```python
from build123d import *

# Parameters (mm, degrees)
F0_R     = 125
F2_DEPTH = 10
F1_R     = 15
F3_DEPTH = 10
F4_R     = 5
F5_R     = 9.544074
F6_DEPTH = 196


with BuildPart() as f2:
    # F0 (on Top) → F2 (new body)
    with BuildSketch(Plane.XY):
        Circle(F0_R)
    extrude(amount=-F2_DEPTH)

    # F1 (on face) → F3 (cut)
    with BuildSketch(Plane.XY):
        with Locations((-42.426407, 42.426407)):
            Circle(F1_R)
        with Locations((0, 60)):
            Circle(F1_R)
        with Locations((42.426407, 42.426407)):
            Circle(F1_R)
        with Locations((60, 0)):
            Circle(F1_R)
        with Locations((42.426407, -42.426407)):
            Circle(F1_R)
        with Locations((0, -60)):
            Circle(F1_R)
        with Locations((-42.426407, -42.426407)):
            Circle(F1_R)
        with Locations((-60, 0)):
            Circle(F1_R)
    extrude(amount=-F3_DEPTH, mode=Mode.SUBTRACT)

    # F4
    f4_edges = [f2.edges().sort_by_distance(p)[0] for p in [
        (-125, 0, 0),
    ]]
    fillet(f4_edges, radius=F4_R)

    # F5 (on face) → F6 (join)
    with BuildSketch(Plane(origin=(0, 0, -10), x_dir=(1, 0, 0), z_dir=(0, 0, -1))):
        with Locations((0, 105.908468)):
            Circle(F5_R)
        with Locations((104.299481, 18.390813)):
            Circle(F5_R)
        with Locations((36.22283, -99.521406)):
            Circle(F5_R)
        with Locations((-91.719424, -52.954234)):
            Circle(F5_R)
    extrude(amount=F6_DEPTH)


solid = f2.part
```
Part model, mm, in its own coordinate system. A direction names the side the tool comes from. Coordinates: 2 decimals unless noted, no trailing zeros. Order: outer loops, then holes, each group sorted by start corner. A loop starts at its lowest first (then second) coordinate and runs counter-clockwise, first axis right, second up. Notation, with made-up numbers: (84.5, 58) - (108.5, 58) arc R19 ccw to (108.5, 90) - close; hole circle Ø10 at (-37, -28.5). An arc over 180 degrees is marked (long way). Return JSON: item names as keys, results as strings. Group by question number.
Item 1: Which spindle directions (+Z, -Z, +X, -X, +Y, -Y) get a long thin tool onto all of the face, cutting with end or side? Do faces 1 (the face through (-2.1, -96.6, -106.6)), 2 (the face through (0, -106, -206)). Say none if no direction does.
Item 2: Cut at C-C (z = -149.5). List the corners of the cut face in (x, y), plus the area to 3 significant figures.
Item 3: Drill centre lines: probe 1 along Y at (x, z) = (0, -7); probe 2 along X at (y, z) = (100, -87.5); probe 3 along Z at (x, y) = (-31.5, 72.5). Where is each one in solid material? Low to high. Write a range as from..to.
Item 4: Cut at B-B (y = 0). List the corners of the cut face in (x, z), plus the area to 3 significant figures.
Item 5: Cut at A-A (x = 0). List the corners of the cut face in (y, z), plus the area to 3 significant figures.
Item 6: Pin check, flat tips, straight feed: pin 1 (18 mm diameter, centred on x = -42.43, y = 42.43, fed in from +Z); pin 2 (2 mm diameter, centred on x = -18, y = -61.5, fed in from +Z); pin 3 (10 mm diameter, centred on x = -98, z = -60, fed in from -Y); pin 4 (12 mm diameter, centred on x = 35.5, z = -166.5, fed in from -Y). Stop position of each tip, or through.
Item 7: Cut at D-D (y = -38.5). State how many separate pieces and enclosed holes the cut face has, plus the area to 3 significant figures.
Item 8: Pull direction X, two halves, no side cores. Call faces 3 (the face through (-92, 53, -206)), 4 (the face through (-44.379, -27.554, -4.93)), 5 (the face through (40.474, -27.554, -4.93)), 6 (the face through (-82.9, 56.6, -106.6)): pulls with the +X half, pulls with the -X half, needs draft (parallel to the pull), parting line crosses it, or undercut.
Check values:
{
 "1": {"face 1": "-Z", "face 2": "-Z, +X, -X, +Y, -Y"},
 "2": {"outline": "circle Ø19.09 at (-91.72, 52.95); circle Ø19.09 at (0, -105.91); circle Ø19.09 at (36.22, 99.52); circle Ø19.09 at (104.3, -18.39)", "area": "1,140 mm2"},
 "3": {"probe 1": "y = -125..-75, -45..45, 75..125", "probe 2": "x = 26.69..45.75", "probe 3": "z = -10..0"},
 "4": {"outline": "(-125, -10) - (-75, -10) - (-75, 0) - (-120, 0) arc R5 ccw to (-125, -5) - close; (-45, -10) - (45, -10) - (45, 0) - (-45, 0) - close; (75, -10) - (125, -10) - (125, -5) arc R5 ccw to (120, 0) - (75, 0) - close", "area": "1,890 mm2"},
 "5": {"outline": "(-125, -10) - (-115.45, -10) - (-115.45, -206) - (-96.36, -206) - (-96.36, -10) - (-75, -10) - (-75, 0) - (-120, 0) arc R5 ccw to (-125, -5) - close; (-45, -10) - (45, -10) - (45, 0) - (-45, 0) - close; (75, -10) - (125, -10) - (125, -5) arc R5 ccw to (120, 0) - (75, 0) - close", "area": "5,630 mm2"},
 "6": {"pin 1": "passes through", "pin 2": "stops at z = 0", "pin 3": "stops at y = 43.5", "pin 4": "stops at y = 89.98"},
 "7": {"separate pieces": "3", "enclosed holes": "0", "area": "1,790 mm2"},
 "8": {"face 3": "needs draft", "face 4": "undercut", "face 5": "undercut", "face 6": "parting line crosses it"}
}
